Source: CAD feature listing. Evaluate the final solid. Frame: model axes, mm. Coordinates: 2 decimals unless noted, no trailing zeros. Loops run counter-clockwise (first coordinate to the right, second up) from the corner with the lowest first, then second, coordinate; pieces in that order, holes last. Notation, with made-up numbers: (87.25, -23) -> (102.25, -23) arc R18 ccw to (102.25, -18) -> close; hole circle Ø3 at (-25.5, 41). An arc over 180 degrees is marked (long way). Answer as a JSON object with one key per item and string values. Group by question number.
from build123d import *

# Parameters (mm, degrees)
EXTRUDE_1_DEPTH                  = 60
SKETCH_2_R                       = 1.4
CUT_EXTRUDE_1_DEPTH              = 61.663003552
SKETCH_3_R                       = 1.4
CUT_EXTRUDE_2_DEPTH              = 61.663003552
PATTERN_LINEAR_1_COUNT           = 4
PATTERN_LINEAR_1_PITCH           = 7
PATTERN_LINEAR_1_COPY_1_SKETCH_R = 1.4
PATTERN_LINEAR_1_COPY_1_DEPTH    = 61.663003552
PATTERN_LINEAR_1_COPY_2_SKETCH_R = 1.4
PATTERN_LINEAR_1_COPY_2_DEPTH    = 61.663003552
PATTERN_LINEAR_1_COPY_3_SKETCH_R = 1.4
PATTERN_LINEAR_1_COPY_3_DEPTH    = 61.663003552
MIRROR_2_COPY_1_SKETCH_R         = 1.4
MIRROR_2_COPY_1_DEPTH            = 61.663003552
MIRROR_2_COPY_2_SKETCH_R         = 1.4
MIRROR_2_COPY_2_DEPTH            = 61.663003552
MIRROR_2_COPY_3_SKETCH_R         = 1.4
MIRROR_2_COPY_3_DEPTH            = 61.663003552
MIRROR_2_COPY_4_SKETCH_R         = 1.4
MIRROR_2_COPY_4_DEPTH            = 61.663003552
MIRROR_2_COPY_5_SKETCH_R         = 1.4
MIRROR_2_COPY_5_DEPTH            = 61.663003552
MIRROR_2_COPY_6_SKETCH_R         = 1.4
MIRROR_2_COPY_6_DEPTH            = 61.663003552
MIRROR_2_COPY_7_SKETCH_R         = 1.4
MIRROR_2_COPY_7_DEPTH            = 61.663003552
EXTRUDE_2_DEPTH                  = 8
EXTRUDE_START                    = -8
EXTRUDE_3_DEPTH                  = 8


with BuildPart() as part:
    # 草图1 → 凸台-拉伸1 (new, symmetric)
    with BuildSketch(Plane.XY):
        with BuildLine():
            Line((-2, -4), (2, -4))
            ThreePointArc((2, -4), (3.414213562, -3.414213562), (4, -2))
            Line((4, -2), (4, 2))
            ThreePointArc((4, 2), (3.414213562, 3.414213562), (2, 4))
            Line((2, 4), (-2, 4))
            ThreePointArc((-2, 4), (-3.414213562, 3.414213562), (-4, 2))
            Line((-4, 2), (-4, -2))
            ThreePointArc((-4, -2), (-3.414213562, -3.414213562), (-2, -4))
        make_face()
    extrude(amount=EXTRUDE_1_DEPTH, both=True)

    # 草图2 → 切除-拉伸1 (cut, through all)
    with BuildSketch(Plane(origin=(4, 0, 0), x_dir=(0, 0, -1), z_dir=(1, 0, 0))):
        Circle(SKETCH_2_R)
    extrude(amount=-CUT_EXTRUDE_1_DEPTH, mode=Mode.SUBTRACT)

    # 草图3 → 切除-拉伸2 (cut, through all)
    with BuildSketch(Plane(origin=(0, 4, 0), x_dir=(1, 0, 0), z_dir=(0, 1, 0))):
        with Locations(Location((0, -54, 0), (0, 0, 270))):
            Circle(SKETCH_3_R)
    cut_extrude_2 = extrude(amount=-CUT_EXTRUDE_2_DEPTH, mode=Mode.SUBTRACT)

    # 镜向1: 切除-拉伸2 across plane
    add(cut_extrude_2.mirror(Plane.XY), mode=Mode.SUBTRACT)

    # 阵列(线性)1: 切除-拉伸2 ×4
    with Locations(*[(0, 0, i * PATTERN_LINEAR_1_PITCH) for i in range(1, PATTERN_LINEAR_1_COUNT)]):
        add(cut_extrude_2, mode=Mode.SUBTRACT)

    # 阵列(线性)1 copy 1 sketch → 阵列(线性)1 copy 1 (cut, through all)
    with BuildSketch(Plane(origin=(0, 4, 7), x_dir=(1, 0, 0), z_dir=(0, 1, 0))):
        with Locations((0, 54)):
            Circle(PATTERN_LINEAR_1_COPY_1_SKETCH_R)
    extrude(amount=-PATTERN_LINEAR_1_COPY_1_DEPTH, mode=Mode.SUBTRACT)

    # 阵列(线性)1 copy 2 sketch → 阵列(线性)1 copy 2 (cut, through all)
    with BuildSketch(Plane(origin=(0, 4, 14), x_dir=(1, 0, 0), z_dir=(0, 1, 0))):
        with Locations((0, 54)):
            Circle(PATTERN_LINEAR_1_COPY_2_SKETCH_R)
    extrude(amount=-PATTERN_LINEAR_1_COPY_2_DEPTH, mode=Mode.SUBTRACT)

    # 阵列(线性)1 copy 3 sketch → 阵列(线性)1 copy 3 (cut, through all)
    with BuildSketch(Plane(origin=(0, 4, 21), x_dir=(1, 0, 0), z_dir=(0, 1, 0))):
        with Locations((0, 54)):
            Circle(PATTERN_LINEAR_1_COPY_3_SKETCH_R)
    extrude(amount=-PATTERN_LINEAR_1_COPY_3_DEPTH, mode=Mode.SUBTRACT)

    # 镜向2 copy 1 sketch → 镜向2 copy 1 (cut, through all)
    with BuildSketch(Plane(origin=(0, 4, -7), x_dir=(1, 0, 0), z_dir=(0, 1, 0))):
        with Locations((0, 54)):
            Circle(MIRROR_2_COPY_1_SKETCH_R)
    extrude(amount=-MIRROR_2_COPY_1_DEPTH, mode=Mode.SUBTRACT)

    # 镜向2 copy 2 sketch → 镜向2 copy 2 (cut, through all)
    with BuildSketch(Plane(origin=(0, 4, -14), x_dir=(1, 0, 0), z_dir=(0, 1, 0))):
        with Locations((0, 54)):
            Circle(MIRROR_2_COPY_2_SKETCH_R)
    extrude(amount=-MIRROR_2_COPY_2_DEPTH, mode=Mode.SUBTRACT)

    # 镜向2 copy 3 sketch → 镜向2 copy 3 (cut, through all)
    with BuildSketch(Plane(origin=(0, 4, -21), x_dir=(1, 0, 0), z_dir=(0, 1, 0))):
        with Locations((0, 54)):
            Circle(MIRROR_2_COPY_3_SKETCH_R)
    extrude(amount=-MIRROR_2_COPY_3_DEPTH, mode=Mode.SUBTRACT)

    # 镜向2 copy 4 sketch → 镜向2 copy 4 (cut, through all)
    with BuildSketch(Plane(origin=(0, 4, -7), x_dir=(1, 0, 0), z_dir=(0, 1, 0))):
        with Locations(Location((0, -54, 0), (0, 0, 270))):
            Circle(MIRROR_2_COPY_4_SKETCH_R)
    extrude(amount=-MIRROR_2_COPY_4_DEPTH, mode=Mode.SUBTRACT)

    # 镜向2 copy 5 sketch → 镜向2 copy 5 (cut, through all)
    with BuildSketch(Plane(origin=(0, 4, -14), x_dir=(1, 0, 0), z_dir=(0, 1, 0))):
        with Locations(Location((0, -54, 0), (0, 0, 270))):
            Circle(MIRROR_2_COPY_5_SKETCH_R)
    extrude(amount=-MIRROR_2_COPY_5_DEPTH, mode=Mode.SUBTRACT)

    # 镜向2 copy 6 sketch → 镜向2 copy 6 (cut, through all)
    with BuildSketch(Plane(origin=(0, 4, -21), x_dir=(1, 0, 0), z_dir=(0, 1, 0))):
        with Locations(Location((0, -54, 0), (0, 0, 270))):
            Circle(MIRROR_2_COPY_6_SKETCH_R)
    extrude(amount=-MIRROR_2_COPY_6_DEPTH, mode=Mode.SUBTRACT)

    # 镜向2 copy 7 sketch → 镜向2 copy 7 (cut, through all)
    with BuildSketch(Plane(origin=(0, 4, 0), x_dir=(1, 0, 0), z_dir=(0, 1, 0))):
        with Locations((0, 54)):
            Circle(MIRROR_2_COPY_7_SKETCH_R)
    extrude(amount=-MIRROR_2_COPY_7_DEPTH, mode=Mode.SUBTRACT)

    # 草图4 → 凸台-拉伸2 (add)
    with BuildSketch(Plane(origin=(0, 4, 0), x_dir=(1, 0, 0), z_dir=(0, 1, 0))):
        with BuildLine():
            Line((-0.979795897, -60), (0.979795897, -60))
            ThreePointArc((0.979795897, -60), (0, -59.6), (-0.979795897, -60))
        make_face()
    extrude(amount=-EXTRUDE_2_DEPTH)

    # 草图5 → 凸台-拉伸3 (add)
    with BuildSketch(Plane.XZ.offset(4).offset(EXTRUDE_START)):
        with BuildLine():
            Line((-0.979795897, -60), (0.979795897, -60))
            ThreePointArc((0.979795897, -60), (0, -59.6), (-0.979795897, -60))
        make_face()
    extrude(amount=EXTRUDE_3_DEPTH)


solid = part.part
1. Pin query (flat end, axial travel): pin 1 Ø1.7 at (x, z) = (0, -33) entering from +Y; pin 2 Ø1 at (y, z) = (3, 6.5) entering from -X. Return the tip coordinate at first contact, or that it passes through.
2. Mould query, pull axis X, two halves, no side actions, for faces 1 (the face through (0.06, 0.06, 31.6)), 2 (the face through (0, 4, 1)), 3 (the face through (4, -1.4, 0.8)), 4 (the face through (-0.18, 0.06, -41.39)). Classes: pulls with the +X half, pulls with the -X half, needs draft (parallel to the pull), parting line crosses it, or undercut.
3. Section query A-A on z = 47. Return loops of the section in (x, y).
4. Section query C-C on z = -24. Return loops of the section in (x, y).
5. Section query B-B on x = 0. State how many separate pieces and enclosed holes the cut face has, then the cut area to 3 significant figures.
6. Ray query, L1, parallel to Y at x = -0.5, z = 0; L2, parallel to Z at x = 3.25, y = -1.25. Return the intervals inside material, ascending.
Solved:
{
 "1": {"pin 1": "through", "pin 2": "x = -3.94"},
 "2": {"face 1": "undercut", "face 2": "needs draft", "face 3": "pulls with the +X half", "face 4": "undercut"},
 "3": {"outline": "(-4, -2) arc R2 ccw to (-2, -4) -> (-1.4, -4) -> (-1.4, 4) -> (-2, 4) arc R2 ccw to (-4, 2) -> close; (1.4, -4) -> (2, -4) arc R2 ccw to (4, -2) -> (4, 2) arc R2 ccw to (2, 4) -> (1.4, 4) -> close"},
 "4": {"outline": "(-4, -2) arc R2 ccw to (-2, -4) -> (2, -4) arc R2 ccw to (4, -2) -> (4, 2) arc R2 ccw to (2, 4) -> (-2, 4) arc R2 ccw to (-4, 2) -> close"},
 "5": {"separate pieces": "9", "enclosed holes": "1", "area": "775 mm^2"},
 "6": {"L1": "-4 to -1.4, 1.4 to 4", "L2": "-60 to -0.63, 0.63 to 60"}
}
